Read the model definition and answer for the solid it produces. Units are mm, in the model's axes. A direction names the side the tool comes from. Give positions to 0.01 mm unless a question says otherwise; leave off trailing zeros. Order: outer loops, then holes, each group sorted by start corner. A loop starts at its lowest first (then second) coordinate and runs counter-clockwise, first axis right, second up. Notation, with made-up numbers: (-16, 39.5) - (20, 39.5) arc R19 ccw to (20, 53.5) - close; hole circle Ø6 at (88.5, 82.5). An arc over 180 degrees is marked (long way). Return JSON: item names as keys, results as strings.
```python
from build123d import *

# Parameters (mm, degrees)
F0_W        = 151.593759656
F0_H        = 151.593759656
F1_DEPTH    = 5
F2_W        = 5.4470277391
F2_H        = 151.593759656
F3_DEPTH    = 70
F4_T1_DEPTH = 366.9308973901
F5_T1_DEPTH = 366.9308973901
F6_W        = 50.1838475466
F6_H        = 51.510296762
F7_DEPTH    = 5
F8_SIZE2    = 4.99999
F8_SIZE     = 3.84999
F9_W        = 73.0733659584
F9_H        = 5.1989573985
F10_DEPTH   = 70
F11_SIZE2   = 70.3308355562
F11_SIZE    = 50
F12_W       = 73.0733659584
F12_H       = 5.0847064704
F13_DEPTH   = 70
F14_SIZE2   = 50
F14_SIZE    = 70.3568348711


# Not quite as in the source:
# - a fillet or chamfer that OpenCascade refuses, or shapes differently, is made with other operations: its cross-section is extruded or revolved along the edge and cut away or added
# - a fillet or chamfer is up to 0.001 mm smaller than in the source, because OpenCascade refuses the exact size


with BuildPart() as f1:
    # F0 (on Top) → F1 (new body)
    with BuildSketch(Plane.XY):
        Rectangle(F0_W, F0_H)
    extrude(amount=F1_DEPTH)

    # F2 (on face) → F3 (join)
    with BuildSketch(Plane.XY.offset(5)):
        Rectangle(F2_W, F2_H)
    extrude(amount=F3_DEPTH)

    # F4: chamfer of 50 x 70 on 1 edges, made by hand

    # F4_s2 → F4_t1 (cut)
    with BuildSketch(Plane.YZ.offset(-183.465448695)):
        Polygon((-75.796879828, 5), (-25.796879828, 75), (-75.796879828, 75), align=None)
    extrude(amount=F4_T1_DEPTH, mode=Mode.SUBTRACT)

    # F5: chamfer of 70 x 50 on 1 edges, made by hand

    # F5_s2 → F5_t1 (cut)
    with BuildSketch(Plane.YZ.offset(-183.465448695)):
        Polygon((75.796879828, 5), (25.796879828, 75), (75.796879828, 75), align=None)
    extrude(amount=F5_T1_DEPTH, mode=Mode.SUBTRACT)

    # F6 (on face) → F7 (join)
    with BuildSketch(Plane.XY.offset(75)):
        Rectangle(F6_W, F6_H)
    extrude(amount=F7_DEPTH)

    # F8 (size 3.85 and 5 in the source; OpenCascade refuses exactly that, so slightly less here)
    f8_edges = [f1.edges().sort_by_distance(p)[0] for p in [
        (25.091924, 0, 80),
        (0, -25.755148, 80),
        (0, 25.755148, 80),
        (-25.091924, 0, 80),
    ]]
    f8_side = f1.faces().sort_by_distance((0, 0, 80))[0]
    chamfer(f8_edges, length=F8_SIZE, length2=F8_SIZE2, reference=f8_side)

    # F9 (on face) → F10 (join)
    with BuildSketch(Plane.XY.offset(5)):
        with Locations((-39.2601968488, 23.0562509969)):
            Rectangle(F9_W, F9_H)
    extrude(amount=F10_DEPTH)

    # F11
    f11_edges = [f1.edges().sort_by_distance(p)[0] for p in [
        (-75.79688, 23.056251, 75),
    ]]
    f11_side = f1.faces().sort_by_distance((-50.444402, 23.056251, 75))[0]
    chamfer(f11_edges, length=F11_SIZE, length2=F11_SIZE2, reference=f11_side)

    # F12 (on face) → F13 (join)
    with BuildSketch(Plane.XY.offset(5)):
        with Locations((39.2601968488, -22.9917196557)):
            Rectangle(F12_W, F12_H)
    extrude(amount=F13_DEPTH)

    # F14
    f14_edges = [f1.edges().sort_by_distance(p)[0] for p in [
        (75.79688, -22.99172, 75),
    ]]
    f14_side = f1.faces().sort_by_distance((75.79688, -74.105559, 2.5))[0]
    chamfer(f14_edges, length=F14_SIZE, length2=F14_SIZE2, reference=f14_side)


solid = f1.part
```
Q1. Consider L1, parallel to Z at x = 16, y = 38; L2, parallel to Y at x = 22, z = 67; L3, parallel to Y at x = -10, z = 68. Determine where each line is inside the solid, lowest interval first.
Values:
{"L1": "z = 0 to 5", "L2": "y = -25.53 to -20.45", "L3": "y = 20.46 to 25.66"}
Q2. For faces 1 (the flat face through (-0.351, 23.857, 77.465)), 2 (the flat face through (-40, -27, 5)), 3 (the flat face through (39, 28, 5)), determine the directions among +Z, -Z, +X, -X, +Y, -Y from which every point of the face is accessible in a straight line to the end or side of a thin tool.
Values:
{"face 1": "+Z, +X, -X, +Y", "face 2": "-X, -Y", "face 3": "+X, +Y"}
Q3. A cutting plane is placed at B-B (y = 62). Write down the section's boundary in (x, z).
Values:
{"outline": "(-75.8, 0) - (75.8, 0) - (75.8, 4.64) - (75.54, 5) - (2.72, 5) - (2.72, 24.32) - (-2.72, 24.32) - (-2.72, 5) - (-75.56, 5) - (-75.8, 4.67) - close"}
Q4. A cutting plane is placed at C-C (z = 41.5). Write down the section's boundary in (x, y), and give its area (3 significant figures).
Values:
{"outline": "(-49.61, 20.46) - (-2.72, 20.46) - (-2.72, -49.73) - (2.72, -49.73) - (2.72, -25.53) - (49.6, -25.53) - (49.6, -20.45) - (2.72, -20.45) - (2.72, 49.73) - (-2.72, 49.73) - (-2.72, 25.66) - (-49.61, 25.66) - close", "area": "1,020 mm²"}
Q5. Given pin 1 (2 mm diameter, centred on x = -3.5, z = 50, fed in from -Y); pin 2 (10 mm diameter, centred on y = -3.5, z = 51.5, fed in from +X); pin 3 (8 mm diameter, centred on x = 51, y = 37.5, fed in from -Z); pin 4 (6 mm diameter, centred on x = 50.5, z = 19, fed in from +Y), each flat-ended and moving along its own axis, determine where each tip first touches the part or whether it passes through.
Values:
{"pin 1": "stops at y = -44.1", "pin 2": "stops at x = 2.72", "pin 3": "stops at z = 0", "pin 4": "stops at y = -20.45"}
Q6. Determine the mould class of faces 4 (the flat face through (31, -20.449, 32)), 5 (the flat face through (-23.19, -0.36, 77.47)), 6 (the flat face through (-75.797, -1, 2)) for opening direction Z: released by +Z, released by -Z, zero draft, split by the parting line, or undercut.
Values:
{"face 4": "undercut", "face 5": "released by +Z", "face 6": "zero draft"}
